```python
from build123d import *

# Parameters (mm, degrees)
SKETCH1_W                   = 9
SKETCH1_H                   = 6
MAIN_BODY_EXT_DEPTH         = 8.3
EMISSION_PATH_EXT_DEPTH     = 9
SKETCH3_R                   = 1.25
EMISSION_AND_GRIN_CUT_DEPTH = 19.125672401
SKETCH4_R                   = 1
DRUM_LENS_CUT_DEPTH         = 7
SKETCH5_W                   = 9
SKETCH5_H                   = 7.3
FILTERSET_CUT1_DEPTH        = 1
FILTERSET_CUT2_DEPTH        = 4
SKETCH10_R                  = 2.5
EMISSION_LENS_CUT_DEPTH     = 8.5
SKETCH15_R                  = 0.795
MAGNETS_CUT_DEPTH           = 0.9
SCREW_HOLES_CUT_DEPTH       = 19.561788707
SCREW_HOLES_CUT_DEPTH_BACK  = 3
SKETCH18_R                  = 0.375
EXTERNAL_FILLET_1_R         = 1.5
CUT_EXTRUDE8_DEPTH          = 12.545128843
CUT_EXTRUDE8_DEPTH_BACK     = 4
SKETCH28_R                  = 1.5
CUT_EXTRUDE9_DEPTH          = 3
CUT_EXTRUDE10_DEPTH         = 0.7
SKETCH29_R                  = 0.375
CUT_EXTRUDE11_DEPTH         = 2.5
SKETCH32_W                  = 2
SKETCH32_H                  = 2.36
CUT_EXTRUDE14_DEPTH         = 0.7
CUT_EXTRUDE16_DEPTH         = 9
CUT_EXTRUDE17_REACH         = 12.329
SKETCH37_R                  = 2


with BuildPart() as part:
    # Sketch1 → Main Body Ext (new body)
    with BuildSketch(Plane(origin=(0, 0, 0), x_dir=(1, 0, 0), z_dir=(0, 1, 0))):
        Rectangle(SKETCH1_W, SKETCH1_H)
    extrude(amount=MAIN_BODY_EXT_DEPTH)

    # Sketch8 → Emission Path Ext (add)
    with BuildSketch(Plane(origin=(0, 8.3, 0), x_dir=(1, 0, 0), z_dir=(0, 1, 0))):
        Polygon((0.25, 3), (1.5, 1.75), (1.5, -3), (-4.5, -3), (-4.5, 3), align=None)
    extrude(amount=EMISSION_PATH_EXT_DEPTH)

    # Sketch3 → Emission and Grin Cut (cut, through all)
    with BuildSketch(Plane.XZ):
        with Locations(Location((-1.5, 0, 0), (0, 0, 270))):
            Circle(SKETCH3_R)
    extrude(amount=-EMISSION_AND_GRIN_CUT_DEPTH, mode=Mode.SUBTRACT)

    # Sketch4 → Drum Lens Cut (cut)
    with BuildSketch(Plane(origin=(4.5, 0, 0), x_dir=(0, 0, -1), z_dir=(1, 0, 0))):
        with Locations((0, 3)):
            Circle(SKETCH4_R)
    extrude(amount=-DRUM_LENS_CUT_DEPTH, mode=Mode.SUBTRACT)

    # Sketch5 → FilterSet Cut1 (cut)
    with BuildSketch(Plane.XY.offset(3)):
        with Locations((0, 4.65)):
            Rectangle(SKETCH5_W, SKETCH5_H)
    extrude(amount=-FILTERSET_CUT1_DEPTH, mode=Mode.SUBTRACT)

    # Sketch6 → FilterSet Cut2 (cut)
    with BuildSketch(Plane.XY.offset(2)):
        with BuildLine():
            Line((2.3, 4.5), (2.3, 1.8))
            ThreePointArc((2.3, 1.8), (2.7, 1.4), (2.3, 1))
            Line((2.3, 1), (1.1, 1))
            ThreePointArc((1.1, 1), (0.7, 1.4), (1.1, 1.8))
            Line((1.1, 1.8), (1.1, 4.5))
            ThreePointArc((1.1, 4.5), (1.7, 5.1), (2.3, 4.5))
        make_face()
        with BuildLine():
            Line((-3.9, 7.9), (-3.9, 7.5))
            ThreePointArc((-3.9, 7.5), (-3.782842712, 7.217157288), (-3.5, 7.1))
            Line((-3.5, 7.1), (0.5, 7.1))
            ThreePointArc((0.5, 7.1), (0.782842712, 7.217157288), (0.9, 7.5))
            Line((0.9, 7.5), (0.9, 7.9))
            ThreePointArc((0.9, 7.9), (0.782842712, 8.182842712), (0.5, 8.3))
            Line((0.5, 8.3), (-3.5, 8.3))
            ThreePointArc((-3.5, 8.3), (-3.782842712, 8.182842712), (-3.9, 7.9))
        make_face()
        with BuildLine():
            Line((0.39411255, 6.591168825), (-3.848528137, 2.348528137))
            ThreePointArc((-3.848528137, 2.348528137), (-3.848528137, 1.5), (-3, 1.5))
            Line((-3, 1.5), (1.242640687, 5.742640687))
            ThreePointArc((1.242640687, 5.742640687), (1.242640687, 6.591168825), (0.39411255, 6.591168825))
        make_face()
    extrude(amount=-FILTERSET_CUT2_DEPTH, mode=Mode.SUBTRACT)

    # Sketch10 → Emission Lens Cut (cut)
    with BuildSketch(Plane(origin=(0, 17.3, 0), x_dir=(1, 0, 0), z_dir=(0, 1, 0))):
        with Locations(Location((-1.5, 0, 0), (0, 0, 270))):
            Circle(SKETCH10_R)
    extrude(amount=-EMISSION_LENS_CUT_DEPTH, mode=Mode.SUBTRACT)

    # Sketch15 → Magnets Cut (cut)
    with BuildSketch(Plane.XZ):
        with Locations(Location((-3.25, -1.875, 0), (0, 0, 270))):
            Circle(SKETCH15_R)
        with Locations(Location((-3.25, 1.875, 0), (0, 0, 270))):
            Circle(SKETCH15_R)
        with Locations(Location((1.5, 0, 0), (0, 0, 270))):
            Circle(SKETCH15_R)
    extrude(amount=-MAGNETS_CUT_DEPTH, mode=Mode.SUBTRACT)

    # Sketch18 → Screw Holes Cut (cut, two sides: drawn at the far end of the back side and taken through both)
    with BuildSketch(Plane.XY.offset(2).offset(-SCREW_HOLES_CUT_DEPTH_BACK)):
        with Locations(Location((-3.5, 4, 0), (0, 0, 180))):
            Circle(SKETCH18_R)
        with Locations(Location((2.5, 6.5, 0), (0, 0, 180))):
            Circle(SKETCH18_R)
        with Locations((3.25, 1)):
            Circle(SKETCH18_R)
    extrude(amount=SCREW_HOLES_CUT_DEPTH + SCREW_HOLES_CUT_DEPTH_BACK, mode=Mode.SUBTRACT)

    # External Fillet 1
    # the kernel refuses this fillet: 1.5 mm, written as the material it takes off along each edge
    with BuildSketch(Plane(origin=(1.5, 8.3, 3), x_dir=(0, 0, -1), z_dir=(0, 1, 0))) as external_fillet_1_piece_1:
        with BuildLine():
            CenterArc((EXTERNAL_FILLET_1_R, EXTERNAL_FILLET_1_R), EXTERNAL_FILLET_1_R, 180, 90)
            Line((0, EXTERNAL_FILLET_1_R), (0, 0))
            Line((0, 0), (EXTERNAL_FILLET_1_R, 0))
        make_face()
    extrude(amount=12.75, mode=Mode.SUBTRACT)
    with BuildSketch(Plane(origin=(-4.5, -3.75, -3), x_dir=(1, 0, 0), z_dir=(0, 1, 0))) as external_fillet_1_piece_2:
        with BuildLine():
            CenterArc((EXTERNAL_FILLET_1_R, -EXTERNAL_FILLET_1_R), EXTERNAL_FILLET_1_R, 90, 90)
            Line((0, -EXTERNAL_FILLET_1_R), (0, 0))
            Line((0, 0), (EXTERNAL_FILLET_1_R, 0))
        make_face()
    extrude(amount=24.8, mode=Mode.SUBTRACT)

    # Sketch28 → Cut-Extrude8 (cut, two sides: drawn at the far end of the back side and taken through both)
    with BuildSketch(Plane(origin=(0, 7.1, 0), x_dir=(1, 0, 0), z_dir=(0, 1, 0)).offset(-CUT_EXTRUDE8_DEPTH_BACK)):
        with Locations(Location((-1.5, 0, 0), (0, 0, 180))):
            Circle(SKETCH28_R)
    extrude(amount=CUT_EXTRUDE8_DEPTH + CUT_EXTRUDE8_DEPTH_BACK, mode=Mode.SUBTRACT)

    # Sketch14 → Cut-Extrude9 (cut)
    with BuildSketch(Plane.XZ):
        Polygon((4.5, -3), (4.5, -2.006698359), (3.837798906, -3), align=None)
    extrude(amount=-CUT_EXTRUDE9_DEPTH, mode=Mode.SUBTRACT)

    # Sketch12 → Cut-Extrude10 (cut)
    with BuildSketch(Plane(origin=(4.5, 0, 0), x_dir=(0, 0, -1), z_dir=(1, 0, 0))):
        with BuildLine():
            Line((1.6, 5.94), (-1.6, 5.94))
            Line((-1.6, 5.94), (-2, 5.94))
            Line((-2, 5.94), (-2, 1.33))
            Line((-2, 1.33), (1.6, 1.33))
            ThreePointArc((1.6, 1.33), (1.882842712, 1.447157288), (2, 1.73))
            Line((2, 1.73), (2, 5.54))
            ThreePointArc((2, 5.54), (1.882842712, 5.822842712), (1.6, 5.94))
        make_face()
    extrude(amount=-CUT_EXTRUDE10_DEPTH, mode=Mode.SUBTRACT)

    # Sketch29 → Cut-Extrude11 (cut)
    with BuildSketch(Plane(origin=(4.5, 0, 0), x_dir=(0, 0, -1), z_dir=(1, 0, 0))):
        with Locations((2, 6.5)):
            Circle(SKETCH29_R)
    extrude(amount=-CUT_EXTRUDE11_DEPTH, mode=Mode.SUBTRACT)

    # Sketch32 → Cut-Extrude14 (cut)
    with BuildSketch(Plane(origin=(4.5, 0, 0), x_dir=(0, 0, -1), z_dir=(1, 0, 0))):
        with Locations((0, 7.12)):
            Rectangle(SKETCH32_W, SKETCH32_H)
    extrude(amount=-CUT_EXTRUDE14_DEPTH, mode=Mode.SUBTRACT)

    # Sketch33 → Cut-Revolve1 (revolve, cut)
    with BuildSketch(Plane.XY, mode=Mode.PRIVATE) as cut_revolve1_sk:
        with BuildLine():
            Line((3.8, 3), (2.3, 3))
            ThreePointArc((2.3, 3), (2.739339828, 4.060660172), (3.8, 4.5))
            Line((3.8, 4.5), (3.8, 3))
        make_face()
    revolve(cut_revolve1_sk.sketch.rotate(Axis((3.8, 3, 0), (-1, 0, 0)), 90), axis=Axis((3.8, 3, 0), (-1, 0, 0)), mode=Mode.SUBTRACT)

    # Sketch36 → Cut-Extrude16 (cut)
    with BuildSketch(Plane(origin=(0, 17.3, 0), x_dir=(1, 0, 0), z_dir=(0, 1, 0))):
        with BuildLine():
            Line((-4.5, -1.5), (-4.5, -3))
            Line((-4.5, -3), (-3, -3))
            ThreePointArc((-3, -3), (-4.060660172, -2.560660172), (-4.5, -1.5))
        make_face()
    extrude(amount=-CUT_EXTRUDE16_DEPTH, mode=Mode.SUBTRACT)

    # Sketch37 → Cut-Extrude17 (cut, up to next)
    with BuildSketch(Plane(origin=(0, 8.8, 0), x_dir=(1, 0, 0), z_dir=(0, 1, 0)), mode=Mode.PRIVATE) as cut_extrude17_sk1:
        with Locations(Location((-1.5, 0, 0), (0, 0, 180))):
            Circle(SKETCH37_R)
    cut_extrude17_tool1 = extrude(cut_extrude17_sk1.sketch, amount=-CUT_EXTRUDE17_REACH, mode=Mode.PRIVATE) & part.part
    add(cut_extrude17_tool1.solids().sort_by_distance((-1.5, 8.8, 0))[0], mode=Mode.SUBTRACT)


solid = part.part
```
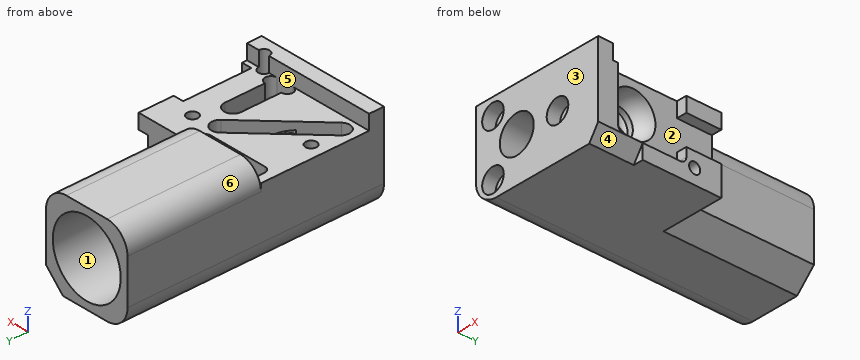
Can you work these out from the model? Positions are in its coordinate system, mm. Face numbers are marked on the shaded views. A direction names the side the tool comes from. Coordinates: 2 decimals unless noted, no trailing zeros. Loops run counter-clockwise (first coordinate to the right, second up) from the corner with the lowest first, then second, coordinate; pieces in that order, holes last.
1) Which directions (+Z, -Z, +X, -X, +Y, -Y) give clear straight access to the entire face, cutting with the end or side of a thin tool? Please do the marked faces 4, 5 and 6.
2) Imagine slicing it at B-B on x = 2.5. List the corners of the cut face in (y, z) for me (3 decimals).
3) Thinking about a two-plate mould opening in Y: for the marked faces 1, 2 and 3, which applies, pulls with the +Y half, pulls with the -Y half, needs draft (parallel to the pull), parting line crosses it, or undercut?
4) Imagine slicing it at A-A on y = 16. List the corners of the cut face in (x, z) for me, plus the area to 3 significant figures.
5) Imagine slicing it at C-C on y = 2.75. State how many separate pieces and enclosed holes the cut face has, plus the area to 3 significant figures.
6) For pin 1 (1.5 mm diameter, centred on x = -1.5, y = 5, fed in from +Z); pin 2 (1.6 mm diameter, centred on y = 3, z = 0, fed in from +X); pin 3 (0.6 mm diameter, centred on x = 2.5, y = 6.5, fed in from +Z), each with a flat end and sliding along its axis, tell me the tip position at first contact or that it passes through.
7) I need wall thicknesses on probe 1 along Y at (x, z) = (-3.5, 0.35) (3 decimals); probe 2 along Z at (x, y) = (0, 15.75); probe 3 along X at (y, z) = (4.6, 0). Which ranges of each line are inside material? Lowest first, please.
Completed:
1. face 4: -Z, +X, -Y
1. face 5: +Z
1. face 6: +Z, -X, +Y
2. outline: (0, -3) - (8.3, -3) - (8.3, 2) - (6.875, 2) - (6.875, -1) - (6.125, -1) - (6.125, 2) - (1.746, 2) - (1.746, -2) - (1.054, -2) - (1.054, 2) - (1, 2) - (1, 3) - (0, 3) - close; hole circle Ø2 at (3, 0); hole circle Ø0.75 at (6.5, -2)
3. face 1: needs draft
3. face 2: undercut
3. face 3: pulls with the -Y half
4. outline: (-4.5, -1.5) arc R1.5 ccw to (-3, -3) - (0.25, -3) - (1.5, -1.75) - (1.5, 1.5) arc R1.5 ccw to (0, 3) - (-3, 3) arc R1.5 ccw to (-4.5, 1.5) - close; hole circle Ø5 at (-1.5, 0)
4. area: 14.1 mm2
5. separate pieces: 3
5. enclosed holes: 0
5. area: 20.1 mm2
6. pin 1: stops at z = 2
6. pin 2: stops at x = -2.82
6. pin 3: stops at z = -1
7. probe 1: y = 0 to 1.329, 2.697 to 3.625, 4.375 to 7.1, 8.3 to 8.8
7. probe 2: z = -3 to -2, 2 to 3
7. probe 3: x = -4.5 to -3, 0.1 to 1.11, 2.29 to 3.8
